Model file for the job. Use its own axes, mm. A direction names the side the tool comes from. Round coordinates to 2 decimals unless told otherwise and drop trailing zeros. Loops run counter-clockwise (first coordinate to the right, second up) from the corner with the lowest first, then second, coordinate; pieces in that order, holes last. Notation, with made-up numbers: (-19.75, 46.25) -> (-3.75, 46.25) arc R20 ccw to (-3.75, 73.25) -> close; hole circle Ø5 at (83, -36). An arc over 180 degrees is marked (long way). Use a Markdown table: item, result.
from build123d import *

# Parameters (mm, degrees)
F0_W     = 57.15
F0_H     = 44.45
F1_DEPTH = 25.4
F3_DEPTH = 12.7
F4_R     = 12.7
F5_DEPTH = 25.4


with BuildPart() as f1:
    # F0 (on Front) → F1 (new body)
    with BuildSketch(Plane.XZ):
        with Locations((28.575, 22.225)):
            Rectangle(F0_W, F0_H)
    extrude(amount=F1_DEPTH)

    # F2 (on face) → F3 (cut)
    with BuildSketch(Plane.XZ.offset(25.4)):
        Polygon((57.15, 44.45), (19.05, 44.45), (44.45, 0), (57.15, 0), align=None)
    extrude(amount=-F3_DEPTH, mode=Mode.SUBTRACT)

    # F4 (on face) → F5 (cut)
    with BuildSketch(Plane(origin=(0, 0, 0), x_dir=(-1, 0, 0), z_dir=(0, 1, 0))):
        with Locations((-25.4, 25.4)):
            Circle(F4_R)
    extrude(amount=-F5_DEPTH, mode=Mode.SUBTRACT)


solid = f1.part
Q1. Band-saw the part on B-B, the plane y = -3. Give the cut face in (x, z), plus the area to 3 significant figures.
Results list:
| item | result |
|---|---|
| outline | (0, 0) -> (57.15, 0) -> (57.15, 44.45) -> (0, 44.45) -> close; hole circle Ø25.4 at (25.4, 25.4) |
| area | 2,030 mm² |
Q2. Band-saw the part on D-D, the plane y = -21.75. Give the cut face in (x, z).
Results list:
| item | result |
|---|---|
| outline | (0, 0) -> (44.45, 0) -> (34.81, 16.87) arc R12.7 cw (long way) to (22.83, 37.84) -> (19.05, 44.45) -> (0, 44.45) -> close |
Q3. Drill centre lines: L1, parallel to Z at x = 25.4, y = -5; L2, parallel to X at y = -12.25, z = 25.4; L3, parallel to Y at x = 31, z = 38. Where is each one in solid material? Low to high. Write a range as from..to.
Results list:
| item | result |
|---|---|
| L1 | z = 0..12.7, 38.1..44.45 |
| L2 | x = 0..12.7, 38.1..57.15 |
| L3 | y = -12.7..0 |
Q4. Pull direction X, two halves, no side cores. Call faces 1 (the face through (13.668, -9.7, 20.536)), 2 (the face through (20.913, -19.139, 41.19)), 3 (the face through (0, -13, 22)), 4 (the face through (28, -13, 0)): released by +X, released by -X, zero draft, split by the parting line, or undercut.
Results list:
| item | result |
|---|---|
| face 1 | undercut |
| face 2 | released by +X |
| face 3 | released by -X |
| face 4 | zero draft |
Q5. Band-saw the part on C-C, the plane z = 24.5. Give the cut face in (x, y).
Results list:
| item | result |
|---|---|
| outline | (0, -25.4) -> (12.73, -25.4) -> (12.73, 0) -> (0, 0) -> close; (38.07, -12.7) -> (57.15, -12.7) -> (57.15, 0) -> (38.07, 0) -> close |
Q6. Band-saw the part on A-A, the plane x = 25.4. Give the cut face in (y, z), plus the area to 3 significant figures.
Results list:
| item | result |
|---|---|
| outline | (-25.4, 0) -> (0, 0) -> (0, 12.7) -> (-25.4, 12.7) -> close; (-12.7, 38.1) -> (0, 38.1) -> (0, 44.45) -> (-12.7, 44.45) -> close |
| area | 403 mm² |
Q7. Tool access for faces 5 (the face through (39.562, -19.139, 8.553)), 6 (the face through (12, -25.4, 18)): list every direction of +Z, -Z, +X, -X, +Y, -Y with a clear straight run to the whole face (end or side of a thin tool).
Results list:
| item | result |
|---|---|
| face 5 | +Z, +X, -Y |
| face 6 | +Z, -Z, +X, -X, -Y |
Q8. Flat gauge pins, fed straight in: pin 1 (4 mm diameter, centred on x = 40.5, z = 39, fed in from +Y); pin 2 (10 mm diameter, centred on y = -19, z = 21, fed in from +X); pin 3 (2 mm diameter, centred on y = -18, z = 15, fed in from +X); pin 4 (1.5 mm diameter, centred on y = -19.5, z = 6, fed in from +X). Where does each tip first touch, or does it go through?
Results list:
| item | result |
|---|---|
| pin 1 | stops at y = 0 |
| pin 2 | stops at x = 35.31 |
| pin 3 | stops at x = 36.45 |
| pin 4 | stops at x = 41.45 |
